Model file for the job. Use its own axes, mm. Face numbers are marked on the shaded views. A direction names the side the tool comes from. Give positions to 0.01 mm unless a question says otherwise; leave off trailing zeros. Order: outer loops, then holes, each group sorted by start corner. A loop starts at its lowest first (then second) coordinate and runs counter-clockwise, first axis right, second up. Notation, with made-up numbers: M 87.5,-20 L 128.5,-20 A33 cw 128.5,16 Z; hole C 4,14.25 d11. An arc over 180 degrees is marked long. Return JSON: item names as keys, results as strings. Group by question number.
1. Pin check, flat tips, straight feed: pin 1 (1 mm diameter, centred on x = -68.5, y = 4.5, fed in from +Z); pin 2 (4 mm diameter, centred on x = -110, y = 2.5, fed in from +Z) (3 decimals); pin 3 (3.5 mm diameter, centred on x = 107.96, y = 0, fed in from -Z). Stop position of each tip, or through.
2. Wall check: probe 1 along X at (y, z) = (-4, 11.5); probe 2 along X at (y, z) = (-1, 1); probe 3 along Z at (x, y) = (5.5, 3.75). Give the ranges that are in metal, low to high. Write a range as [from, to].
3. Two-plate mould, pull along X, no slides. Class the marked faces 1, 2 and 3: released by +X, released by -X, zero draft, split by the parting line, or undercut.
4. Slice it at B-B on x = 24. List the corners of the cut face in (y, z).
5. 3-axis set-ups, long thin cutter, end or side, ignore diameter. For the marked faces 4 and 5: which of +Z, -Z, +X, -X, +Y, -Y reach the whole face in a straight line?
6. Slice it at A-A on y = 0. List the corners of the cut face in (x, z) (1 decimal), then the cut area to 3 significant figures.
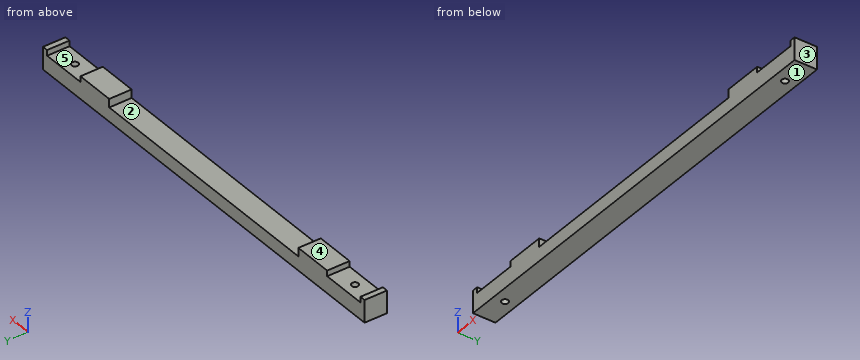
from build123d import *

# Parameters (mm, degrees)
SKETCH1_W           = 247.9294
SKETCH1_H           = 12.7
BOSS_EXTRUDE1_DEPTH = 12.7
SKETCH2_W           = 25.654
SKETCH2_H           = 21.428464986
CUT_EXTRUDE1_DEPTH  = 3.175
SKETCH3_W           = 145.8214
SKETCH3_H           = 22.473236176
CUT_EXTRUDE2_DEPTH  = 4.7625
CUT_EXTRUDE3_START  = -9.525
SKETCH4_R           = 1.905
CUT_EXTRUDE3_DEPTH  = 9.525


with BuildPart() as part:
    # Sketch1 → Boss-Extrude1 (new body)
    with BuildSketch(Plane.XY):
        Rectangle(SKETCH1_W, SKETCH1_H)
    extrude(amount=BOSS_EXTRUDE1_DEPTH)

    # Sketch2 → Cut-Extrude1 (cut)
    with BuildSketch(Plane.XY.offset(12.7)):
        with Locations((-107.9627, 0)):
            Rectangle(SKETCH2_W, SKETCH2_H)
        with Locations((107.9627, 0)):
            Rectangle(SKETCH2_W, SKETCH2_H)
    extrude(amount=-CUT_EXTRUDE1_DEPTH, mode=Mode.SUBTRACT)

    # Sketch3 → Cut-Extrude2 (cut)
    with BuildSketch(Plane.XY.offset(12.7)):
        Rectangle(SKETCH3_W, SKETCH3_H)
    extrude(amount=-CUT_EXTRUDE2_DEPTH, mode=Mode.SUBTRACT)

    # Sketch4 → Cut-Extrude3 (cut)
    with BuildSketch(Plane.XY.offset(9.525).offset(CUT_EXTRUDE3_START)):
        with Locations((-107.9627, 0)):
            Circle(SKETCH4_R)
        with Locations((107.9627, 0)):
            Circle(SKETCH4_R)
    extrude(amount=CUT_EXTRUDE3_DEPTH, mode=Mode.SUBTRACT)


solid = part.part
Result:
{
 "1": {"pin 1": "stops at z = 7.94", "pin 2": "stops at z = 9.525", "pin 3": "passes through"},
 "2": {"probe 1": "x = [-123.96, -120.79], [-95.14, -72.91], [72.91, 95.14], [120.79, 123.96]", "probe 2": "x = [-123.96, -109.58], [-106.34, 106.34], [109.58, 123.96]", "probe 3": "z = [0, 7.94]"},
 "3": {"face 1": "zero draft", "face 2": "undercut", "face 3": "released by +X"},
 "4": {"outline": "M -6.35,0 L 6.35,0 L 6.35,7.94 L -6.35,7.94 Z"},
 "5": {"face 4": "+Z, +X, -X, +Y, -Y", "face 5": "+Z, +Y, -Y"},
 "6": {"outline": "M -124,0 L -109.9,0 L -109.9,9.5 L -120.8,9.5 L -120.8,12.7 L -124,12.7 Z; M -106.1,0 L 106.1,0 L 106.1,9.5 L 95.1,9.5 L 95.1,12.7 L 72.9,12.7 L 72.9,7.9 L -72.9,7.9 L -72.9,12.7 L -95.1,12.7 L -95.1,9.5 L -106.1,9.5 Z; M 109.9,0 L 124,0 L 124,12.7 L 120.8,12.7 L 120.8,9.5 L 109.9,9.5 Z", "area": "2,220 mm2"}
}
